Design review of the part built by this model. Coordinates are the model's own, in mm. Face numbers are marked on the shaded views. A direction names the side the tool comes from. Coordinates: 2 decimals unless noted, no trailing zeros. Write each loop counter-clockwise with the first axis right and the second up, starting at its lowest first coordinate (ties: lowest second). Pieces come first, ordered by that corner, then holes. Notation, with made-up numbers: M 53.5,12 L 85.5,12 A32 cw 85.5,49 Z; hole C 35,60 d5. An arc over 180 degrees is marked long. One line per question, with ' | ' between items.
from build123d import *

# Parameters (mm, degrees)
F2_R     = 12.7
F3_R     = 5.08
F4_R     = 4.3688
F5_DEPTH = 12.7
F6_COUNT = 4


with BuildPart() as f1:
    # F0 (on Right) → F1 (revolve)
    with BuildSketch(Plane.YZ):
        Polygon((0, 72.5043), (0, 35.2425), (5.08, 30.1625), (14.9352, 30.1625), (14.9352, 21.336), (16.9672, 21.336), (16.9672, 18.0086), (22.0218, 18.0086), (22.0218, 35.4337260178), (22.7838, 36.1957260178), (22.7838, 40.005), (46.9646, 40.005), (46.9646, 50.8), (11.557, 57.0433152021), (11.557, 114.4524), (23.4784016177, 114.4524), (31.5722, 114.4524), (31.5722, 118.2624), (26.797, 118.2624), (26.797, 121.5898), (4.7625, 119.6620310435), (4.7625, 90.4875), (3.175, 88.9), (3.175, 72.5043), align=None)
    revolve(axis=Axis((0, 65.5152718432, 0), (0, 1, 0)))

    # F2
    f2_edges = [f1.edges().sort_by_distance(p)[0] for p in [
        (0, 11.557, -114.4524),
    ]]
    fillet(f2_edges, radius=F2_R)

    # F3
    f3_edges = [f1.edges().sort_by_distance(p)[0] for p in [
        (0, 11.557, -57.043315),
    ]]
    fillet(f3_edges, radius=F3_R)

    # F4 (on face) → F5 (join)
    with BuildSketch(Plane(origin=(0, 26.797, 0), x_dir=(-1, 0, 0), z_dir=(0, 1, 0))):
        with BuildLine():
            Line((104.775, 61.6950471192), (104.775, 94.7858482647))
            ThreePointArc((104.775, 94.7858482647), (99.9053493469, 99.9053493469), (94.7858482647, 104.775))
            Line((94.7858482647, 104.775), (61.6950471192, 104.775))
            ThreePointArc((61.6950471192, 104.775), (85.9769721031, 85.9769721031), (104.775, 61.6950471192))
        make_face()
        with Locations((93.6625, 93.6625)):
            Circle(F4_R, mode=Mode.SUBTRACT)
        with BuildLine():
            Line((104.775, 54.8470111197), (104.775, 61.6950471192))
            ThreePointArc((104.775, 61.6950471192), (85.9769721031, 85.9769721031), (61.6950471192, 104.775))
            Line((61.6950471192, 104.775), (54.8470111197, 104.775))
            ThreePointArc((54.8470111197, 104.775), (83.6241449994, 83.6241449994), (104.775, 54.8470111197))
        make_face()
    extrude(amount=-F5_DEPTH)

    # F6: F1 ×4 about axis
    f6_axis = Axis((0, 16.9672, 0), (0, 1, 0))


with BuildPart() as f1_1:
    add(f1.part)
    for i in range(1, F6_COUNT):
        add(f1.part.rotate(f6_axis, i * 360 / F6_COUNT))


solid = f1_1.part
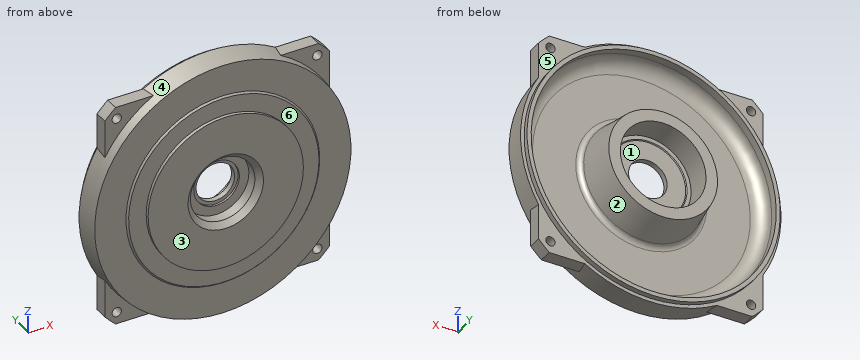
1. Take a section at A-A (y = 38). Write out the cut boundary in (x, z) (3 decimals).
Answer sheet:
outline: C 0,0 d104.761; hole C 0,0 d80.01
2. Tool access review of the marked faces 5 and 6: name each direction out of +Z, -Z, +X, -X, +Y, -Y from which nothing blocks a thin tool from reaching the whole face with its end or side.
Answer sheet:
face 5: +Y | face 6: -Y
3. Draft analysis for pull direction Z (two halves, no side actions). For the marked faces 1, 2, 3 and 4, state which applies: pulls with the +Z half, pulls with the -Z half, needs draft (parallel to the pull), parting line crosses it, or undercut.
Answer sheet:
face 1: undercut | face 2: undercut | face 3: needs draft | face 4: parting line crosses it
4. Insertion check: pin 1 Ø13.5 at (x, z) = (-81.5, -76) entering from -Y; pin 2 Ø10 at (y, z) = (5, 34) entering from +X; pin 3 Ø2 at (x, y) = (21.5, 26) entering from -Z. Each pin has a flat end and moves straight along its axis. Give the tip position at first contact, or say it passes through.
Answer sheet:
pin 1: y = 4.76 | pin 2: x = 116.19 | pin 3: z = -119.8
5. To check wall thickness, follow line 1 along X through (y, z) = (29.5, 0) (3 decimals); line 2 along X through (y, z) = (28.5, 36); line 3 along X through (y, z) = (24, 41). State the ranges of each line that lie inside material, in increasing order. Write a range as [from, to].
Answer sheet:
line 1: [-118.262, -114.452], [-53.879, -40.005], [40.005, 53.879], [114.452, 118.262] | line 2: [-112.65, -108.64], [-40.32, -17.45], [17.45, 40.32], [108.64, 112.65] | line 3: [-114.21, -106.85], [-36.43, 36.43], [106.85, 114.21]
